```python
from build123d import *

# Parameters (mm, degrees)
SKETCH1_W           = 150
SKETCH1_H           = 80
BOSS_EXTRUDE1_DEPTH = 60


with BuildPart() as part:
    # Sketch1 → Boss-Extrude1 (new body)
    with BuildSketch(Plane(origin=(0, 0, 0), x_dir=(1, 0, 0), z_dir=(0, 1, 0))):
        Rectangle(SKETCH1_W, SKETCH1_H)
    extrude(amount=BOSS_EXTRUDE1_DEPTH)

    # Sketch2 → Cut-Revolve1 (revolve, cut)
    with BuildSketch(Plane.XY):
        Polygon((-40, 60), (-70, 60), (-55, 50), (-55, 10), (-40, 10), align=None)
    cut_revolve1 = revolve(axis=Axis((-40, 10, 0), (0, 1, 0)), mode=Mode.SUBTRACT)

    # Mirror1: Cut-Revolve1 across plane
    add(cut_revolve1.mirror(Plane(origin=(0, 0, 0), x_dir=(0, 0, 1), z_dir=(1, 0, 0))), mode=Mode.SUBTRACT)


solid = part.part
```
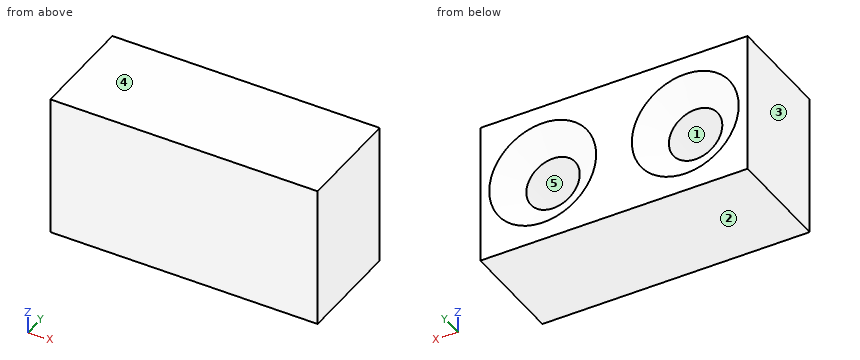
Geometry: final body of the model. Coordinates: model frame, mm. Face numbers are marked on the shaded views. A direction names the side the tool comes from. Round coordinates to 2 decimals unless told otherwise and drop trailing zeros. Order: outer loops, then holes, each group sorted by start corner. A loop starts at its lowest first (then second) coordinate and runs counter-clockwise, first axis right, second up. Notation, with made-up numbers: M 85,20 L 121,20 A28 ccw 121,39 Z; hole C 67,87 d5. An arc over 180 degrees is marked long. One line per item, written item: value.
(1) Pin query (flat end, axial travel): P1, Ø24, axis at x = 39.5, z = -2.5, coming from the +Y side. Return the tip coordinate at first contact, or that it passes through.
Result sheet:
P1: y = 10
(2) Pull-direction query (Z, two-part tool) for the marked faces 1, 2 and 3; classes: pulls with the +Z half, pulls with the -Z half, needs draft (parallel to the pull), parting line crosses it, or undercut.
Result sheet:
face 1: undercut
face 2: pulls with the -Z half
face 3: needs draft
(3) Cut plane B-B (y = 19). Return the cut outline in (x, z).
Result sheet:
outline: M -75,-40 L 75,-40 L 75,40 L -75,40 Z; hole C -40,0 d30; hole C 40,0 d30
(4) Cut plane C-C (x = 40). Return the cut outline in (y, z), and give its area (3 significant figures).
Result sheet:
outline: M 0,-40 L 60,-40 L 60,-30 L 50,-15 L 10,-15 L 10,15 L 50,15 L 60,30 L 60,40 L 0,40 Z
area: 3,150 mm2
(5) Line query: probe 1 along Z at (x, y) = (40, 30); probe 2 along X at (y, z) = (47.5, 6); probe 3 along Z at (x, y) = (34.5, 46.5). Output: solid intervals per line, ascending. Write a range as [from, to].
Result sheet:
probe 1: [-40, -15], [15, 40]
probe 2: [-75, -53.75], [-26.25, 26.25], [53.75, 75]
probe 3: [-40, -13.96], [13.96, 40]
(6) Reachability of the marked faces 4 and 5 from +Z, -Z, +X, -X, +Y, -Y: full face, straight path, thin tool, end or side. Return the list, or none.
Result sheet:
face 4: +Z, +X, -X, +Y, -Y
face 5: +Y
(7) Cut plane A-A (z = 0). Return the cut outline in (x, y), and give its area (3 significant figures).
Result sheet:
outline: M -75,0 L 75,0 L 75,60 L 70,60 L 55,50 L 55,10 L 25,10 L 25,50 L 10,60 L -10,60 L -25,50 L -25,10 L -55,10 L -55,50 L -70,60 L -75,60 Z
area: 5,700 mm2
